```python
from build123d import *

# Parameters (mm, degrees)
SKETCH1_R           = 125
BOSS_EXTRUDE1_DEPTH = 0.8


with BuildPart() as part:
    # Sketch1 → Boss-Extrude1 (new body)
    with BuildSketch(Plane(origin=(0, 0, 0), x_dir=(1, 0, 0), z_dir=(0, 1, 0))):
        with Locations(Location((0, 0, 0), (0, 0, 270))):
            Circle(SKETCH1_R)
        with BuildLine():
            ThreePointArc((17.637470301, 95.583703669), (35.39721968, 96.175428091), (53.159818023, 95.676493311))
            add(Edge.make_bspline(
                [(53.159818023, 95.676493311), (56.08234597, 94.996231289), (58.564200991, 93.194770615), (60.361809914, 90.792161995)],
                knots=[0, 0, 0, 0, 1, 1, 1, 1], degree=3))
            add(Edge.make_bspline(
                [(60.350685033, -90.839559126), (99.288183814, -0.082759064), (60.361809914, 90.792161995)],
                knots=[1.080613073, 1.080613073, 1.080613073, 2.054120599, 2.054120599, 2.054120599], degree=2, weights=[1, 0.88385597, 1]))
            add(Edge.make_bspline(
                [(60.350685033, -90.839559126), (58.536259011, -93.25472766), (56.008057905, -95.005350463), (53.084387141, -95.765172879)],
                knots=[0, 0, 0, 0, 1, 1, 1, 1], degree=3))
            ThreePointArc((53.084387141, -95.765172879), (35.358173243, -96.209231493), (17.637146794, -95.591923789))
            add(Edge.make_bspline(
                [(17.637146794, -95.591923789), (14.078918858, -94.177841771), (11.966771187, -90.615205857), (12.239909507, -86.796042408)],
                knots=[0, 0, 0, 0, 1, 1, 1, 1], degree=3))
            add(Edge.make_bspline(
                [(12.239909507, -86.796042408), (17.237181475, -72.608584217), (24.453254999, -59.238409711), (31.894828879, -30.090174015), (33.746605648, -15.047383971), (33.791634635, 15.036244417), (31.895103774, 30.080327703), (24.444131359, 59.226605128), (16.862561087, 72.474291436), (12.25464212, 86.792942903)],
                knots=[0, 0, 0, 0, 0.25, 0.25, 0.5, 0.5, 0.75, 0.75, 1, 1, 1, 1], degree=3))
            add(Edge.make_bspline(
                [(12.25464212, 86.792942903), (11.86155894, 90.601686389), (14.119358115, 94.07243666), (17.637470301, 95.583703669)],
                knots=[0, 0, 0, 0, 1, 1, 1, 1], degree=3))
        make_face(mode=Mode.SUBTRACT)
        with BuildLine():
            add(Edge.make_bspline(
                [(-63.760090493, -86.796042408), (-58.762818525, -72.608584217), (-51.546745001, -59.238409711), (-44.105171121, -30.090174015), (-42.253394352, -15.047383971), (-42.208365365, 15.036244417), (-44.104896226, 30.080327703), (-51.555868641, 59.226605128), (-59.137438913, 72.474291436), (-63.74535788, 86.792942903)],
                knots=[0, 0, 0, 0, 0.25, 0.25, 0.5, 0.5, 0.75, 0.75, 1, 1, 1, 1], degree=3))
            add(Edge.make_bspline(
                [(-63.74535788, 86.792942903), (-64.13844106, 90.601686389), (-61.880641885, 94.07243666), (-58.362529699, 95.583703669)],
                knots=[0, 0, 0, 0, 1, 1, 1, 1], degree=3))
            ThreePointArc((-58.362529699, 95.583703669), (-40.60278032, 96.175428091), (-22.840181977, 95.676493311))
            add(Edge.make_bspline(
                [(-22.840181977, 95.676493311), (-19.91765403, 94.996231289), (-17.435799009, 93.194770615), (-15.638190086, 90.792161995)],
                knots=[0, 0, 0, 0, 1, 1, 1, 1], degree=3))
            add(Edge.make_bspline(
                [(-15.649314967, -90.839559126), (23.288183814, -0.082759064), (-15.638190086, 90.792161995)],
                knots=[1.080613073, 1.080613073, 1.080613073, 2.054120599, 2.054120599, 2.054120599], degree=2, weights=[1, 0.88385597, 1]))
            add(Edge.make_bspline(
                [(-15.649314967, -90.839559126), (-17.463740989, -93.25472766), (-19.991942095, -95.005350463), (-22.915612859, -95.765172879)],
                knots=[0, 0, 0, 0, 1, 1, 1, 1], degree=3))
            ThreePointArc((-22.915612859, -95.765172879), (-40.641826757, -96.209231493), (-58.362853206, -95.591923789))
            add(Edge.make_bspline(
                [(-58.362853206, -95.591923789), (-61.921081142, -94.177841771), (-64.033228813, -90.615205857), (-63.760090493, -86.796042408)],
                knots=[0, 0, 0, 0, 1, 1, 1, 1], degree=3))
        make_face(mode=Mode.SUBTRACT)
    extrude(amount=BOSS_EXTRUDE1_DEPTH)


solid = part.part
```
Input: part model. Units: mm. Frame: model coordinates. Coordinates: 2 decimals unless noted, no trailing zeros. Write each loop counter-clockwise with the first axis right and the second up, starting at its lowest first coordinate (ties: lowest second). Pieces come first, ordered by that corner, then holes. Notation, with made-up numbers: M 74.25,65.25 L 125.25,65.25 A16 ccw 125.25,76.25 Z; hole C 43,36.25 d10. An arc over 180 degrees is marked long. Use one line per item in the form item = value.
Q1. Section C-C (x = 86). Return loops of the section in (y, z).
Answer below:
outline = M 0,-90.71 L 0.8,-90.71 L 0.8,90.71 L 0,90.71 Z
Q2. Material intervals for probe 1 along X at (y, z) = (0.4, 0); probe 2 along X at (y, z) = (0.7, -3); probe 3 along Z at (x, y) = (18, 0.45), sorted ascending. Write a range as from..to.
Answer below:
probe_1 = -125..-42.23, 2.62..33.77, 78.62..125
probe_2 = -124.96..-42.25, 2.6..33.75, 78.6..124.96
probe_3 = -123.7..-95.61, -71.8..72.25, 95.62..123.7
Q3. Section B-B (z = 58). Count the separate pieces of the cut face and the enclosed holes in it, plus the area to 3 significant figures.
Answer below:
separate_pieces = 3
enclosed_holes = 0
area = 101 mm²
Q4. Section A-A (x = 48). Return loops of the section in (y, z).
Answer below:
outline = M 0,-115.42 L 0.8,-115.42 L 0.8,-95.93 L 0,-95.93 Z; M 0,96 L 0.8,96 L 0.8,115.42 L 0,115.42 Z
